```python
from build123d import *

# Parameters (mm, degrees)
SKETCH_1_W                  = 320
SKETCH_1_H                  = 100
EXTRUDE_1_DEPTH             = 3
HOLE_WIZARD_4_0_4_1_D       = 4
HOLE_WIZARD_4_2_4_2_1_D     = 4.2
PATTERN_LINEAR_1_COUNT      = 2
PATTERN_LINEAR_1_PITCH      = 95
PATTERN_LINEAR_1_COUNT_DIR2 = 2
PATTERN_LINEAR_1_PITCH_DIR2 = 25
CUT_EXTRUDE_1_DEPTH         = 3
SKETCH_8_W                  = 24
SKETCH_8_H                  = 45
CUT_EXTRUDE_6_DEPTH         = 3
PATTERN_LINEAR_2_COUNT      = 2
PATTERN_LINEAR_2_PITCH      = 60
PATTERN_LINEAR_2_COPY_1_D   = 4
HOLE_WIZARD_3_0_3_1_D       = 3
CUT_EXTRUDE_8_DEPTH         = 3
FILLET_1_R                  = 12
PATTERN_LINEAR_3_COUNT      = 2
PATTERN_LINEAR_3_PITCH      = 80
PATTERN_LINEAR_3_COPY_1_D   = 4
FILLET_2_R                  = 5
CUT_EXTRUDE_9_DEPTH         = 3
FILLET_3_R                  = 2
CUT_EXTRUDE_10_DEPTH        = 10


with BuildPart() as part:
    # 草图1 → 凸台-拉伸1 (new body)
    with BuildSketch(Plane.XY):
        Rectangle(SKETCH_1_W, SKETCH_1_H)
    extrude(amount=EXTRUDE_1_DEPTH)

    # Ø4.0 (4) 直径孔1 (through all)
    with Locations(Plane(origin=(0, 0, 0), x_dir=(-1, 0, 0), z_dir=(0, 0, -1))):
        with Locations((108, -40)):
            hole_wizard_4_0_4_1 = Hole(HOLE_WIZARD_4_0_4_1_D / 2)

    # 镜向1: Ø4.0 (4) 直径孔1 across plane
    add(hole_wizard_4_0_4_1.mirror(Plane(origin=(0, 0, 0), x_dir=(0, 0, 1), z_dir=(1, 0, 0))), mode=Mode.SUBTRACT)

    # Ø4.2 (4.2) 直径孔1 (through all)
    with Locations(Plane(origin=(0, 0, 0), x_dir=(-1, 0, 0), z_dir=(0, 0, -1))):
        with Locations((47.5, 0)):
            hole_wizard_4_2_4_2_1 = Hole(HOLE_WIZARD_4_2_4_2_1_D / 2)

    # 阵列(线性)1: Hole Wizard 4.2 _4.2_ _1 2 × 2
    with Locations(*[(i * PATTERN_LINEAR_1_PITCH, j * PATTERN_LINEAR_1_PITCH_DIR2, 0) for i in range(PATTERN_LINEAR_1_COUNT) for j in range(PATTERN_LINEAR_1_COUNT_DIR2) if (i, j) != (0, 0)]):
        add(hole_wizard_4_2_4_2_1, mode=Mode.SUBTRACT)

    # 草图6 → 切除-拉伸1 (cut)
    with BuildSketch(Plane(origin=(0, 0, 0), x_dir=(-1, 0, 0), z_dir=(0, 0, -1))):
        Polygon((0, -50), (0, -10), (70, -10), (95, -50), align=None)
    cut_extrude_1 = extrude(amount=-CUT_EXTRUDE_1_DEPTH, mode=Mode.SUBTRACT)

    # 镜向2: 切除-拉伸1 across plane
    add(cut_extrude_1.mirror(Plane(origin=(0, -50, 3), x_dir=(0, 0, 1), z_dir=(1, 0, 0))), mode=Mode.SUBTRACT)

    # 草图8 → 切除-拉伸6 (cut)
    with BuildSketch(Plane(origin=(0, 0, 0), x_dir=(-1, 0, 0), z_dir=(0, 0, -1))):
        with Locations((-133, -12.5)):
            Rectangle(SKETCH_8_W, SKETCH_8_H)
    cut_extrude_6 = extrude(amount=-CUT_EXTRUDE_6_DEPTH, mode=Mode.SUBTRACT)

    # 镜向4: 切除-拉伸6 across plane
    add(cut_extrude_6.mirror(Plane(origin=(0, 0, 0), x_dir=(0, 0, 1), z_dir=(1, 0, 0))), mode=Mode.SUBTRACT)

    # 阵列(线性)2: Ø4.0 (4) 直径孔1 ×2
    with Locations(*[(0, i * PATTERN_LINEAR_2_PITCH, 0) for i in range(1, PATTERN_LINEAR_2_COUNT)]):
        add(hole_wizard_4_0_4_1, mode=Mode.SUBTRACT)

    # 阵列(线性)2 copy 1 (through all)
    with Locations(Plane(origin=(0, 60, 0), x_dir=(1, 0, 0), z_dir=(0, 0, -1))):
        with Locations((108, 40)):
            Hole(PATTERN_LINEAR_2_COPY_1_D / 2)

    # Ø3.0 (3) 直径孔1 (through all)
    with Locations(Plane.XY.offset(3)):
        with Locations((-152.5, -40), (-152.5, -12)):
            hole_wizard_3_0_3_1 = Hole(HOLE_WIZARD_3_0_3_1_D / 2)

    # 草图11 → 切除-拉伸8 (cut)
    with BuildSketch(Plane.XY.offset(3)):
        Polygon((-118, 50), (-160, 50), (-160, 20), align=None)
    cut_extrude_8 = extrude(amount=-CUT_EXTRUDE_8_DEPTH, mode=Mode.SUBTRACT)

    # 镜向6: 切除-拉伸8 across plane
    add(cut_extrude_8.mirror(Plane(origin=(0, 0, 0), x_dir=(0, 0, 1), z_dir=(1, 0, 0))), mode=Mode.SUBTRACT)

    # 镜向7: Ø3.0 (3) 直径孔1 across plane
    add(hole_wizard_3_0_3_1.mirror(Plane(origin=(0, 0, 0), x_dir=(0, 0, 1), z_dir=(1, 0, 0))), mode=Mode.SUBTRACT)

    # 圆角1
    fillet_1_edges = [part.edges().sort_by_distance(p)[0] for p in [
        (145, -35, 1.5),
        (121, -35, 1.5),
        (145, 10, 1.5),
        (121, 10, 1.5),
        (-145, -35, 1.5),
        (-121, -35, 1.5),
        (-145, 10, 1.5),
        (-121, 10, 1.5),
    ]]
    fillet(fillet_1_edges, radius=FILLET_1_R - 0.0001)  # a hair under: the kernel refuses the full size

    # 阵列(线性)3: Ø4.0 (4) 直径孔1 ×2
    with Locations(*[(0, i * PATTERN_LINEAR_3_PITCH, 0) for i in range(1, PATTERN_LINEAR_3_COUNT)]):
        add(hole_wizard_4_0_4_1, mode=Mode.SUBTRACT)

    # 阵列(线性)3 copy 1 (through all)
    with Locations(Plane(origin=(0, 80, 0), x_dir=(1, 0, 0), z_dir=(0, 0, -1))):
        with Locations((108, 40)):
            Hole(PATTERN_LINEAR_3_COPY_1_D / 2)

    # 圆角2
    fillet_2_edges = [part.edges().sort_by_distance(p)[0] for p in [
        (-160, 20, 1.5),
        (-118, 50, 1.5),
        (160, 20, 1.5),
        (118, 50, 1.5),
        (-95, -50, 1.5),
        (-70, -10, 1.5),
        (95, -50, 1.5),
        (70, -10, 1.5),
        (160, -50, 1.5),
        (-160, -50, 1.5),
    ]]
    fillet(fillet_2_edges, radius=FILLET_2_R)

    # 草图12 → 切除-拉伸9 (cut)
    with BuildSketch(Plane(origin=(0, 0, 0), x_dir=(-1, 0, 0), z_dir=(0, 0, -1))):
        Polygon((-89.16731107, -17.567353927), (-78.38158698, -1.676376149), (-89.16731107, 14.034356584), align=None)
        Polygon((-90.804111964, 39.84100352), (-62.022726086, 39.84100352), (-62.022726086, -0.778396903), align=None)
    cut_extrude_9 = extrude(amount=-CUT_EXTRUDE_9_DEPTH, mode=Mode.SUBTRACT)

    # 镜向8: 切除-拉伸9 across plane
    add(cut_extrude_9.mirror(Plane(origin=(0, 0, 0), x_dir=(0, 0, 1), z_dir=(1, 0, 0))), mode=Mode.SUBTRACT)

    # 圆角3
    fillet_3_edges = [part.edges().sort_by_distance(p)[0] for p in [
        (89.16731107, -17.567353927, 1.5),
        (89.16731107, 14.034356584, 1.5),
        (78.38158698, -1.676376149, 1.5),
        (62.022726086, -0.778396903, 1.5),
        (90.804111964, 39.84100352, 1.5),
        (62.022726086, 39.84100352, 1.5),
        (-89.16731107, 14.034356584, 1.5),
        (-89.16731107, -17.567353927, 1.5),
        (-78.38158698, -1.676376149, 1.5),
        (-90.804111964, 39.84100352, 1.5),
        (-62.022726086, -0.778396903, 1.5),
        (-62.022726086, 39.84100352, 1.5),
    ]]
    fillet(fillet_3_edges, radius=FILLET_3_R)

    # 草图13 → 切除-拉伸10 (cut)
    with BuildSketch(Plane.XY.offset(3)):
        Polygon((-23.094010768, 20), (-11.547005384, 0), (11.547005384, 0), (23.094010768, 20), (11.547005384, 40), (-11.547005384, 40), align=None)
    extrude(amount=-CUT_EXTRUDE_10_DEPTH, mode=Mode.SUBTRACT)


solid = part.part
```
Check sheet for the modelled part. Datum: model origin and axes. Units: mm. A direction names the side the tool comes from. Round coordinates to 2 decimals unless told otherwise and drop trailing zeros. Loops run counter-clockwise (first coordinate to the right, second up) from the corner with the lowest first, then second, coordinate; pieces in that order, holes last. Notation, with made-up numbers: (87.25, 49.5) -> (114.25, 49.5) arc R18 cw to (114.25, 75.5) -> close; hole circle Ø4 at (30, 8.5). An arc over 180 degrees is marked (long way). Answer in a Markdown table with one row per item.
Q1. Sectioned sample at B-B on z = 1.55. Give the number of separate pieces and of enclosed holes in the cut face, then the cut area to 3 significant figures.
Data:
| item | result |
|---|---|
| separate pieces | 1 |
| enclosed holes | 21 |
| area | 19,200 mm^2 |
Q2. Sectioned sample at D-D on x = 58.5. Enter the section's corners in (y, z), then the cut area to 3 significant figures.
Data:
| item | result |
|---|---|
| outline | (-10, 0) -> (50, 0) -> (50, 3) -> (-10, 3) -> close |
| area | 180 mm^2 |
Q3. Release check for a two-part mould opening along X. For faces 1 (the face through (-38, 12, 3)), 2 (the face through (17.4, 29.86, 1.52)), 3 (the face through (-139, 35, 2)), 4 (the face through (139, 35, 2)) record: released by +X, released by -X, zero draft, split by the parting line, or undercut.
Data:
| item | result |
|---|---|
| face 1 | zero draft |
| face 2 | undercut |
| face 3 | released by -X |
| face 4 | released by +X |
Q4. Go/stop test with a flat-tipped pin: P1, Ø4, axis at x = 152.5, y = -40, coming from the -Z side. Record where the tip stops, or that it passes through.
Data:
| item | result |
|---|---|
| P1 | stops at z = 0 |
Q5. Sectioned sample at A-A on x = -4. Enter the section's corners in (y, z), then the cut area to 3 significant figures.
Data:
| item | result |
|---|---|
| outline | (-10, 0) -> (0, 0) -> (0, 3) -> (-10, 3) -> close; (40, 0) -> (50, 0) -> (50, 3) -> (40, 3) -> close |
| area | 60.0 mm^2 |
Q6. Set-up check for faces 5 (the face through (17.24, 9.86, 1.52)), 6 (the face through (-82.346, -29.753, 1.479)): record each of +Z, -Z, +X, -X, +Y, -Y from which the full face is reachable in a straight line by a thin tool's end or side.
Data:
| item | result |
|---|---|
| face 5 | +Z, -Z |
| face 6 | +Z, -Z, -Y |
Q7. Sectioned sample at C-C on x = 127. Enter the section's corners in (y, z).
Data:
| item | result |
|---|---|
| outline | (-50, 0) -> (-33.39, 0) -> (-33.39, 3) -> (-50, 3) -> close; (8.39, 0) -> (43.57, 0) -> (43.57, 3) -> (8.39, 3) -> close |
Q8. Thickness scan on L1, parallel to Y at x = -108, z = 1.4; L2, parallel to Y at x = 47, z = 2.85; L3, parallel to Y at x = 84.5, z = 0.65. Record the ranges inside material, lowest first.
Data:
| item | result |
|---|---|
| L1 | y = -50 to -42, -38 to 18, 22 to 38, 42 to 50 |
| L2 | y = -10 to -2.04, 2.04 to 22.96, 27.04 to 50 |
| L3 | y = -33.2 to -10.69, 7.24 to 30.94, 39.84 to 50 |
